Geometry: final body of the model. Coordinates: model frame, mm. A direction names the side the tool comes from. Round coordinates to 2 decimals unless told otherwise and drop trailing zeros. Loops run counter-clockwise (first coordinate to the right, second up) from the corner with the lowest first, then second, coordinate; pieces in that order, holes last. Notation, with made-up numbers: (49.25, -24.5) - (86.25, -24.5) arc R34 cw to (86.25, 14.5) - close; hole circle Ø7 at (-11.5, -10). An arc over 180 degrees is marked (long way). Answer as CSV lines item,"result".
from build123d import *

# Parameters (mm, degrees)
EXTRUDE_1_DEPTH             = 24
EXTRUDE_1_DEPTH_BACK        = 6
EXTRUDE_2_DEPTH             = 18
HOLE_WIZARD_M41_D           = 3.3
HOLE_WIZARD_M41_DEPTH       = 11.5
HOLE_WIZARD_M41_CSINK_D     = 4.05
HOLE_WIZARD_M41_CSINK_ANGLE = 120
HOLE_WIZARD_M41_TIP         = 0.991420021
HOLE_WIZARD_M61_D           = 5
HOLE_WIZARD_M61_DEPTH       = 17
HOLE_WIZARD_M61_CSINK_D     = 6.05
HOLE_WIZARD_M61_CSINK_ANGLE = 120
HOLE_WIZARD_M61_TIP         = 1.502151548


with BuildPart() as part:
    # Эскиз1 → Бобышка-Вытянуть1 (new, two sides: drawn at the far end of the back side and taken through both)
    with BuildSketch(Plane.XY.offset(-EXTRUDE_1_DEPTH_BACK)):
        with BuildLine():
            Line((28.5, 9), (40, 9))
            Line((40, 9), (40, 0))
            Line((40, 0), (0, 0))
            Line((0, 0), (0, 9))
            Line((0, 9), (11.5, 9))
            ThreePointArc((11.5, 9), (20, 0.5), (28.5, 9))
        make_face()
    extrude(amount=EXTRUDE_1_DEPTH + EXTRUDE_1_DEPTH_BACK)

    # Эскиз3 → Бобышка-Вытянуть2 (add)
    with BuildSketch(Plane.XY):
        with BuildLine():
            Line((11.5, 9), (14, 9))
            ThreePointArc((14, 9), (20, 3), (26, 9))
            Line((26, 9), (28.5, 9))
            ThreePointArc((28.5, 9), (20, 0.5), (11.5, 9))
        make_face()
    extrude(amount=EXTRUDE_2_DEPTH)

    # Отверстие обработанное метчиком M41
    with Locations(Plane.XZ):
        with Locations((35, 19), (35, -1), (5, 19), (5, -1)):
            CounterSinkHole(HOLE_WIZARD_M41_D / 2, HOLE_WIZARD_M41_CSINK_D / 2, depth=HOLE_WIZARD_M41_DEPTH, counter_sink_angle=HOLE_WIZARD_M41_CSINK_ANGLE)
            with Locations((0, 0, -(HOLE_WIZARD_M41_DEPTH + HOLE_WIZARD_M41_TIP / 2))):  # 118° drill point
                Cone(0, HOLE_WIZARD_M41_D / 2, HOLE_WIZARD_M41_TIP, mode=Mode.SUBTRACT)

    # Отверстие обработанное метчиком M61
    with Locations(Plane(origin=(0, 9, 0), x_dir=(-1, 0, 0), z_dir=(0, 1, 0))):
        with Locations((-32.5, 9), (-7.5, 9)):
            CounterSinkHole(HOLE_WIZARD_M61_D / 2, HOLE_WIZARD_M61_CSINK_D / 2, depth=HOLE_WIZARD_M61_DEPTH, counter_sink_angle=HOLE_WIZARD_M61_CSINK_ANGLE)
            with Locations((0, 0, -(HOLE_WIZARD_M61_DEPTH + HOLE_WIZARD_M61_TIP / 2))):  # 118° drill point
                Cone(0, HOLE_WIZARD_M61_D / 2, HOLE_WIZARD_M61_TIP, mode=Mode.SUBTRACT)


solid = part.part
(1) Section A-A (z = 9). Output: boundary loops of the cut face in (x, y) (3 decimals).
Findings below:
outline,"(0, 0) - (5, 0) - (5, 8.697) - (4.475, 9) - (0, 9) - close; (10, 0) - (30, 0) - (30, 8.697) - (29.475, 9) - (26, 9) arc R6 cw to (14, 9) - (10.525, 9) - (10, 8.697) - close; (35, 0) - (40, 0) - (40, 9) - (35.525, 9) - (35, 8.697) - close"
(2) Section C-C (y = 6). Output: boundary loops of the cut face in (x, z), and give its area (3 significant figures).
Findings below:
outline,"(0, -6) - (12.05, -6) - (12.05, 0) - (14.8, 0) - (14.8, 18) - (12.05, 18) - (12.05, 24) - (0, 24) - close; (25.2, 0) - (27.95, 0) - (27.95, -6) - (40, -6) - (40, 24) - (27.95, 24) - (27.95, 18) - (25.2, 18) - close; hole circle Ø3.3 at (5, -1); hole circle Ø3.3 at (5, 19); hole circle Ø5 at (7.5, 9); hole circle Ø5 at (32.5, 9); hole circle Ø3.3 at (35, -1); hole circle Ø3.3 at (35, 19)"
area,"749 mm2"
(3) Draft query along Z for faces 1 (the face through (24.7, 1.6, 24)), 2 (the face through (5.215, 4.67, 20.636)), 3 (the face through (4, 9, 9)). Return one class per face: pulls with the +Z half, pulls with the -Z half, needs draft (parallel to the pull), parting line crosses it, or undercut.
Findings below:
face 1,"pulls with the +Z half"
face 2,"undercut"
face 3,"needs draft"
(4) Access query for faces 4 (the face through (36.65, 4.67, -0.93)), 5 (the face through (19.813, 0.502, 20.958)), 6 (the face through (20, 2, 0)). Directions: +Z, -Z, +X, -X, +Y, -Y. A direction counts if a zero-diameter tool reaches every point of the face in a straight line with its end or side. Return the directions, or none.
Findings below:
face 4,"+Y, -Y"
face 5,"+Z, +Y"
face 6,"-Z, +Y"
(5) Section D-D (y = 2.5). Output: boundary loops of the cut face in (x, z).
Findings below:
outline,"(0, -6) - (14.52, -6) - (14.52, 0) - (25.48, 0) - (25.48, -6) - (40, -6) - (40, 24) - (25.48, 24) - (25.48, 18) - (14.52, 18) - (14.52, 24) - (0, 24) - close; hole circle Ø3.3 at (5, -1); hole circle Ø3.3 at (5, 19); hole circle Ø5 at (7.5, 9); hole circle Ø5 at (32.5, 9); hole circle Ø3.3 at (35, -1); hole circle Ø3.3 at (35, 19)"
(6) Pin query (flat end, axial travel): P1, Ø4, axis at x = 35, z = -1, coming from the -Y side; P2, Ø4, axis at x = 15, y = 5.5, coming from the +Z side; P3, Ø4.5, axis at x = 35, z = 19, coming from the +Y side. Return the tip coordinate at first contact, or that it passes through.
Findings below:
P1,"y = 0.01"
P2,"z = 18"
P3,"y = 9"
(7) Section B-B (x = 32.5). Output: boundary loops of the cut face in (y, z) (3 decimals).
Findings below:
outline,"(0, -6) - (9, -6) - (9, 5.975) - (8.697, 6.5) - (0, 6.5) - close; (0, 11.5) - (8.697, 11.5) - (9, 12.025) - (9, 24) - (0, 24) - close"
(8) Material intervals for line 1 along X through (y, z) = (3.75, 19); line 2 along X through (y, z) = (1, 10.5); line 3 along X through (y, z) = (8.5, 7.75), sorted ascending.
Findings below:
line 1,"0 to 3.35, 6.65 to 13.32, 26.68 to 33.35, 36.65 to 40"
line 2,"0 to 5.5, 9.5 to 30.5, 34.5 to 40"
line 3,"0 to 5.33, 9.67 to 14.02, 25.98 to 30.33, 34.67 to 40"
